Read the model definition and answer for the solid it produces. Units are mm, in the model's axes. Face numbers are marked on the shaded views. A direction names the side the tool comes from. Round coordinates to 2 decimals unless told otherwise and drop trailing zeros. Loops run counter-clockwise (first coordinate to the right, second up) from the corner with the lowest first, then second, coordinate; pieces in that order, holes last. Notation, with made-up numbers: (7.25, 2) - (53.25, 2) arc R26 ccw to (53.25, 36) - close; hole circle Ø3 at (44, 25.25). An arc over 180 degrees is marked (long way). Use CSV: the item, a comma, the result in double quotes. Start each with the question number.
1. Consider line 1 along Y through (x, z) = (20, 8.75); line 2 along X through (y, z) = (28.5, 1.5); line 3 along Y through (x, z) = (44, 5.5). Determine where each line is inside the solid, lowest interval first.
2. Determine the mould class of the marked faces 1, 2, 3 and 4 for opening direction X: +X half, -X half, draft (parallel to the pull), parting line (faces both ways), or undercut.
3. Given pin 1 Ø1.5 at (y, z) = (27.5, 4) entering from -X; pin 2 Ø2 at (x, z) = (16.5, 18.5) entering from +Y; pin 3 Ø16 at (x, y) = (20, 20) entering from +Z; pin 4 Ø8 at (x, y) = (38, 24) entering from +Z, each flat-ended and moving along its own axis, determine where each tip first touches the part or whether it passes through.
4. Find section D-D (z = 21). Give the vertices of the cut face in (x, y).
5. Find section B-B (x = 23). Give the vertices of the cut face in (y, z).
6. Find section C-C (x = 52). Give the vertices of the cut face in (y, z), and give its area (3 significant figures).
7. A tool of negligible diameter and unlimited length cuts with its end or side. For the marked faces 5, 6 and 7, from which of +Z, -Z, +X, -X, +Y, -Y can it reach the whole face along a straight path? Write none if from no direction.
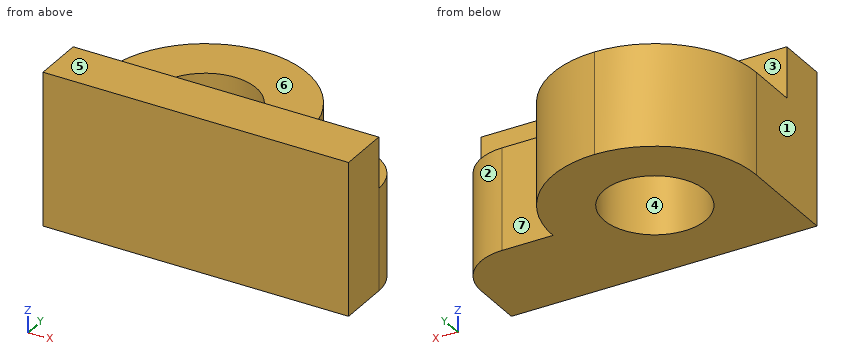
Autodesk Inventor part; units mm, degrees
ref_plane "YZ Plane" through (0, 0, 0) normal (1, 0, 0) x (0, 1, 0)
ref_plane "XZ Plane" through (0, 0, 0) normal (0, 1, 0) x (-1, 0, 0)
ref_plane "XY Plane" through (0, 0, 0) normal (0, 0, 1) x (1, 0, 0)
sketch "草圖1" plane through (0, 0, 0) normal (0, 0, 1) x (1, 0, 0)
  line L0 (0, 0) -> (60, 0)
  line L1 (60, 0) -> (60, 20)
  line L2 (60, 20) -> (0, 20)
  line L3 (0, 20) -> (0, 0)
  line L4 (0, 20) -> (40, 20)
  line L5 (40, 20) -> (40, 40)
  line L6 (40, 40) -> (0, 40)
  line L7 (0, 40) -> (0, 20)
  dimension "d0" = 20
  dimension "d1" = 20
  dimension "d2" = 60
  dimension "d3" = 40
extrude "擠出1" add sketch "草圖1" along normal blind 20
fillet "圓角1" radius 20 2 edges at (40, 40, 10) (0, 40, 10)
fillet "圓角2" radius 10 1 edges at (60, 20, 10)
sketch "草圖2" plane through (0, 0, 20) normal (0, 0, 1) x (1, 0, 0)
  line L0 (60, 0) -> (60, 10)
  line L1 (0, 20) -> (0, 0)
  line L2 (60, 10) -> (0, 10)
  line L3 (0, 10) -> (0, 0)
  line L4 (0, 0) -> (60, 0)
  line L5 (60, 0) -> (60, 10)
extrude "擠出2" add sketch "草圖2" along normal blind 10
sketch "草圖3" plane through (0, 0, 20) normal (0, 0, 1) x (1, 0, 0)
  arc A0 (40, 20) -> (0, 20) centre (20, 20) ccw
  circle A1 centre (20, 20) radius 10
  line L0 (0, 10) -> (60, 10)
  point P0 (0, 0)
extrude "擠出3" cut sketch "草圖3" against normal through all
properties part number "4"
Filled sheet:
1,line 1,"y = 0 to 10, 30 to 40"
1,line 2,"x = 1.9 to 14.73, 25.27 to 38.1"
1,line 3,"y = 0 to 20"
2,face 1,"-X half"
2,face 2,"+X half"
2,face 3,"draft"
2,face 4,"undercut"
3,pin 1,"stops at x = 1.17"
3,pin 2,"stops at y = 39.84"
3,pin 3,"passes through"
3,pin 4,"stops at z = 20"
4,outline,"(0, 0) - (60, 0) - (60, 10) - (0, 10) - close"
5,outline,"(0, 0) - (10.46, 0) - (10.46, 20) - (10, 20) - (10, 30) - (0, 30) - close; (29.54, 0) - (39.77, 0) - (39.77, 20) - (29.54, 20) - close"
6,outline,"(0, 0) - (19.8, 0) - (19.8, 20) - (10, 20) - (10, 30) - (0, 30) - close"
6,area,"496 mm²"
7,face 5,"+Z, +X, -X, +Y, -Y"
7,face 6,"+Z, +X, -X, +Y"
7,face 7,"+Z, -Z, +X, +Y"
